The listing builds one solid part. Answer for the finished solid, in the listing's coordinates (mm). Face numbers are marked on the shaded views. A direction names the side the tool comes from. Coordinates: 2 decimals unless noted, no trailing zeros. Order: outer loops, then holes, each group sorted by start corner. A loop starts at its lowest first (then second) coordinate and runs counter-clockwise, first axis right, second up. Notation, with made-up numbers: (-22.5, 21.25) -> (14.5, 21.25) arc R15 cw to (14.5, 43.25) -> close; hole circle Ø7 at (36.25, -21). An arc over 180 degrees is marked (long way). Return JSON: item names as keys, results as strings.
```python
from build123d import *

# Parameters (mm, degrees)
PAD001_DEPTH      = 16
PAD001_DEPTH_BACK = 16
SKETCH014_W       = 15
SKETCH014_H       = 6
POCKET_DEPTH      = 28.001
SKETCH012_R       = 5.15
POCKET001_DEPTH   = 55.001
SKETCH013_R       = 1.75
POCKET002_DEPTH   = 7
SKETCH008_W       = 7.907674
SKETCH008_H       = 14
POCKET003_DEPTH   = 33
SKETCH007_R       = 1.75
POCKET004_DEPTH   = 17.001
SKETCH015_W       = 50.47
SKETCH015_H       = 40
POCKET005_DEPTH   = 2
FILLET_R          = 2
FILLET001_R       = 1
FILLET002_R       = 1
FILLET003_R       = 1
FILLET004_R       = 2


with BuildPart() as part:
    # Sketch005 → Pad001 (new body, two sides)
    with BuildSketch(Plane.YZ) as pad001_sk:
        Polygon((0, -20), (0, 25), (3, 25), (3, 35), (-25, 35), (-25, 25), (-14, 25), (-14, -20), align=None)
    extrude(amount=PAD001_DEPTH)
    extrude(pad001_sk.sketch, amount=-PAD001_DEPTH_BACK)

    # Sketch014 (on Face5 of Pad001) → Pocket (cut, through all)
    with BuildSketch(Plane(origin=(0, -25, 0), x_dir=(0, 0, -1), z_dir=(0, -1, 0))):
        with Locations((-20.5, -5)):
            Rectangle(SKETCH014_W, SKETCH014_H)
    extrude(amount=-POCKET_DEPTH, mode=Mode.SUBTRACT)

    # Sketch012 → Pocket001 (cut, through all)
    with BuildSketch(Plane(origin=(0, 0, 35), x_dir=(0, -1, 0), z_dir=(0, 0, 1))):
        with Locations((13, -5)):
            Circle(SKETCH012_R)
    extrude(amount=-POCKET001_DEPTH, mode=Mode.SUBTRACT)

    # Sketch013 → Pocket002 (cut)
    with BuildSketch(Plane(origin=(0, 0, 35), x_dir=(0, -1, 0), z_dir=(0, 0, 1))):
        with Locations((4, -5)):
            Circle(SKETCH013_R)
        with Locations((22, -5)):
            Circle(SKETCH013_R)
    extrude(amount=-POCKET002_DEPTH, mode=Mode.SUBTRACT)

    # Sketch008 (on Face9 of Pocket002) → Pocket003 (cut)
    with BuildSketch(Plane.YX.offset(20)):
        with Locations((-10.953837, -7)):
            Rectangle(SKETCH008_W, SKETCH008_H)
    extrude(amount=-POCKET003_DEPTH, mode=Mode.SUBTRACT)

    # Sketch007 (on Face21 of Pocket003) → Pocket004 (cut, through all)
    with BuildSketch(Plane(origin=(0, -14, 0), x_dir=(0, 0, -1), z_dir=(0, -1, 0))):
        with Locations((-6, 10)):
            Circle(SKETCH007_R)
        with Locations((14, 10)):
            Circle(SKETCH007_R)
        with Locations((-6, -10)):
            Circle(SKETCH007_R)
        with Locations((14, -10)):
            Circle(SKETCH007_R)
    extrude(amount=-POCKET004_DEPTH, mode=Mode.SUBTRACT)

    # Sketch015 (on Face1 of Pocket004) → Pocket005 (cut)
    with BuildSketch(Plane.ZX):
        with Locations((-4.235, 0)):
            Rectangle(SKETCH015_W, SKETCH015_H)
    extrude(amount=-POCKET005_DEPTH, mode=Mode.SUBTRACT)

    # Fillet
    fillet_edges = [part.edges().sort_by_distance(p)[0] for p in [
        (16, 3, 30),
        (-16, 3, 30),
        (-16, -25, 30),
        (16, -25, 30),
    ]]
    fillet(fillet_edges, radius=FILLET_R)

    # Fillet001
    fillet001_edges = [part.edges().sort_by_distance(p)[0] for p in [
        (0.05198, -14, 2.5),
        (-10.05198, -14, 19),
    ]]
    fillet(fillet001_edges, radius=FILLET001_R)

    # Fillet002
    fillet002_edges = [part.edges().sort_by_distance(p)[0] for p in [
        (-2, -25, 26.5),
        (-8, -25, 26.5),
    ]]
    fillet(fillet002_edges, radius=FILLET002_R)

    # Fillet003
    fillet003_edges = [part.edges().sort_by_distance(p)[0] for p in [
        (-16, 0, 23),
        (16, 0, 23),
    ]]
    fillet(fillet003_edges, radius=FILLET003_R)

    # Fillet004
    fillet004_edges = [part.edges().sort_by_distance(p)[0] for p in [
        (16, -14, 2.5),
    ]]
    fillet(fillet004_edges, radius=FILLET004_R)


solid = part.part
```
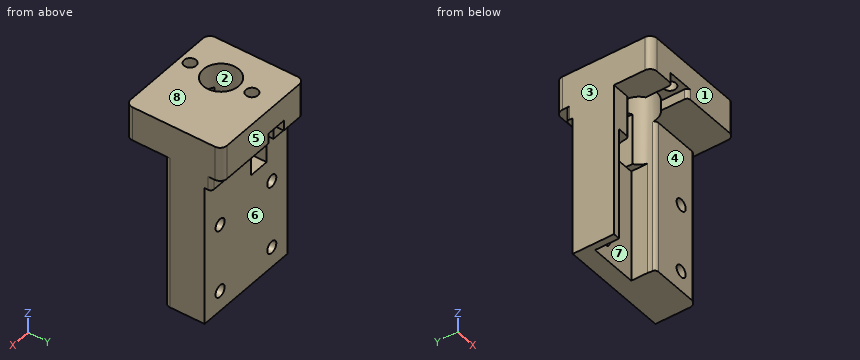
Item 1: Find the intervals of material crossed by probe 1 along X at (y, z) = (-8.25, 6); probe 2 along X at (y, z) = (-6.25, -14); probe 3 along Y at (x, z) = (-8, 31), in increasing order.
Answer list:
{"probe 1": "-16 to -14, 0 to 8.25, 11.75 to 16", "probe 2": "-16 to -11.75, -8.25 to 8.25, 11.75 to 16", "probe 3": "-25 to -17.19, -8.81 to 3"}
Item 2: The part is cut by section A-A on z = 17. Determine the outline of the cut face in (x, y), plus the area to 3 significant figures.
Answer list:
{"outline": "(-16, -14) -> (-11.15, -14) arc R1 ccw to (-10.15, -13) arc R5.15 cw to (-8, -8.81) -> (-8, -2) -> (-16, -2) -> close; (-2, -8.81) arc R5.15 cw to (0.15, -13) arc R1 ccw to (1.15, -14) -> (14, -14) arc R2 ccw to (16, -12) -> (16, -2) -> (-2, -2) -> close", "area": "294 mm2"}
Item 3: Which of the six approach directions +Z, -Z, +X, -X, +Y, -Y give full straight-line access (tool end or side, diameter ignored) to the marked faces 4, 5, 6, 7 and 8?
Answer list:
{"face 4": "-Z, +X, -X, -Y", "face 5": "+Z, -Z, +X, -X, +Y", "face 6": "-Z, +X, -X, +Y", "face 7": "-Z, -Y", "face 8": "+Z, +X, -X, +Y, -Y"}
Item 4: Flat-ended cylindrical pins translate along their axes: pin 1 (4 mm diameter, centred on x = 5, y = -20, fed in from -Z); pin 2 (2 mm diameter, centred on x = 5.5, z = 23.5, fed in from +Y); pin 3 (3 mm diameter, centred on x = -11.5, y = -10.5, fed in from -Z); pin 4 (6 mm diameter, centred on x = -1, y = -11, fed in from -Z). Find the tip coordinate at first contact, or state that the pin passes through.
Answer list:
{"pin 1": "z = 25", "pin 2": "y = 0", "pin 3": "z = 13", "pin 4": "z = -20"}
Item 5: The part is cut by section B-B on y = -4. Determine the outline of the cut face in (x, z), plus the area to 3 significant figures.
Answer list:
{"outline": "(-16, -20) -> (16, -20) -> (16, 35) -> (-3.25, 35) -> (-3.25, 28) -> (-2, 28) -> (-2, 13) -> (-8, 13) -> (-8, 28) -> (-6.75, 28) -> (-6.75, 35) -> (-16, 35) -> close; hole circle Ø3.5 at (-10, -14); hole circle Ø3.5 at (-10, 6); hole circle Ø3.5 at (10, -14); hole circle Ø3.5 at (10, 6)", "area": "1,610 mm2"}
Item 6: Determine the mould class of the marked faces 1, 2 and 3 for opening direction X: pulls with the +X half, pulls with the -X half, needs draft (parallel to the pull), parting line crosses it, or undercut.
Answer list:
{"face 1": "needs draft", "face 2": "undercut", "face 3": "pulls with the -X half"}
Item 7: The part is cut by section C-C on y = -22. Determine the outline of the cut face in (x, z), plus the area to 4 significant figures.
Answer list:
{"outline": "(-16, 25) -> (-8, 25) -> (-8, 28) -> (-6.75, 28) -> (-6.75, 35) -> (-16, 35) -> close; (-3.25, 28) -> (-2, 28) -> (-2, 25) -> (16, 25) -> (16, 35) -> (-3.25, 35) -> close", "area": "277.5 mm2"}
Item 8: The part is cut by section D-D on x = 10. Determine the outline of the cut face in (y, z), plus the area to 3 significant figures.
Answer list:
{"outline": "(-25, 25) -> (-14, 25) -> (-14, 7.75) -> (-2, 7.75) -> (-2, 21) -> (0, 21) -> (0, 25) -> (3, 25) -> (3, 35) -> (-25, 35) -> close; (-14, -20) -> (-2, -20) -> (-2, -15.75) -> (-14, -15.75) -> close; (-14, -12.25) -> (-2, -12.25) -> (-2, 4.25) -> (-14, 4.25) -> close", "area": "744 mm2"}
